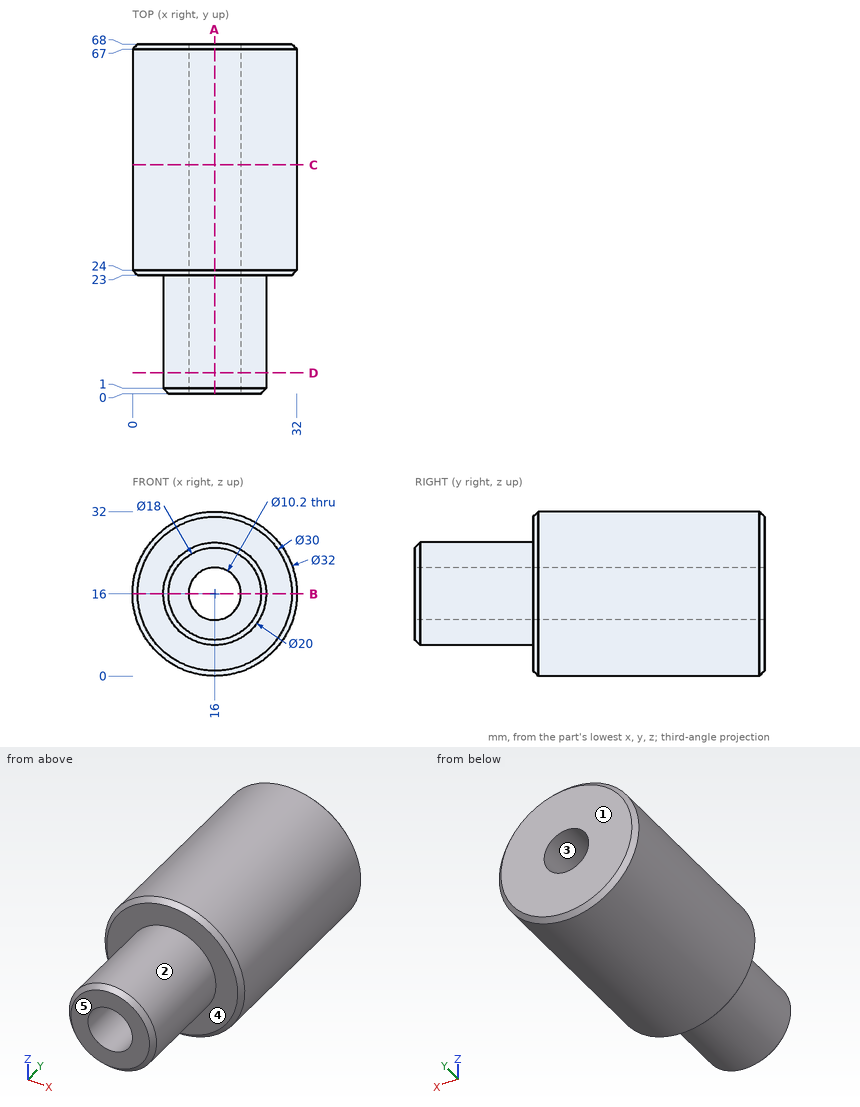
Source: three-view drawing plus pictorial views. Frame: mm from the lowest corner of the part. A direction names the side the tool comes from. Round coordinates to 2 decimals unless told otherwise and drop trailing zeros. Loops run counter-clockwise (first coordinate to the right, second up) from the corner with the lowest first, then second, coordinate; pieces in that order, holes last.
Item 1: Section D-D, the plane y = 4. Output: boundary loops of the cut face in (x, z).
Checked values:
outline: circle Ø20 at (16, 16); hole circle Ø10.2 at (16, 16)
Item 2: Section B-B, the plane z = 16. Output: boundary loops of the cut face in (x, y).
Checked values:
outline: (0, 24) - (1, 23) - (6, 23) - (6, 1) - (7, 0) - (10.9, 0) - (10.9, 68) - (1, 68) - (0, 67) - close; (21.1, 0) - (25, 0) - (26, 1) - (26, 23) - (31, 23) - (32, 24) - (32, 67) - (31, 68) - (21.1, 68) - close
Item 3: Section A-A, the plane x = 16. Output: boundary loops of the cut face in (y, z).
Checked values:
outline: (0, 7) - (1, 6) - (23, 6) - (23, 1) - (24, 0) - (67, 0) - (68, 1) - (68, 10.9) - (0, 10.9) - close; (0, 21.1) - (68, 21.1) - (68, 31) - (67, 32) - (24, 32) - (23, 31) - (23, 26) - (1, 26) - (0, 25) - close
Item 4: Reachability of the marked faces 4 and 5 from +Z, -Z, +X, -X, +Y, -Y: full face, straight path, thin tool, end or side. Return the list, or none.
Checked values:
face 4: -Y
face 5: +Z, -Z, +X, -X, -Y
Item 5: Mould query, pull axis Z, two halves, no side actions, for the marked faces 1, 2 and 3. Classes: released by +Z, released by -Z, zero draft, split by the parting line, or undercut.
Checked values:
face 1: zero draft
face 2: split by the parting line
face 3: undercut
Item 6: Section C-C, the plane y = 44.5. Output: boundary loops of the cut face in (x, z), plus the area to 3 significant figures.
Checked values:
outline: circle Ø32 at (16, 16); hole circle Ø10.2 at (16, 16)
area: 723 mm2
Item 7: Contact query for flat-ended pins moving along their axis: P1, Ø10, axis at y = 47.5, z = 25.5, coming from the +X side; P2, Ø12, axis at x = 8.5, y = 37.5, coming from the +Z side; P3, Ø8, axis at y = 43, z = 20.5, coming from the -X side. Output: stop coordinate, or through.
Checked values:
P1: stops at x = 31.35
P2: stops at z = 31.93
P3: stops at x = 0.01
Item 8: Line query: L1, parallel to Z at x = 16, y = 20; L2, parallel to Y at x = 17.5, z = 29; L3, parallel to Z at x = 17, y = 49.5. Output: solid intervals per line, ascending.
Checked values:
L1: z = 6 to 10.9, 21.1 to 26
L2: y = 23 to 68
L3: z = 0.03 to 11, 21 to 31.97
